Here's how the part is built. I have some questions about the finished solid (model axes, mm). A direction names the side the tool comes from. Coordinates: 2 decimals unless noted, no trailing zeros. Write each loop counter-clockwise with the first axis right and the second up, starting at its lowest first coordinate (ties: lowest second). Pieces come first, ordered by that corner, then holes.
```python
from build123d import *

# Parameters (mm, degrees)
PROFILE_R   = 2.5
PROFILE_R_2 = 1


with BuildPart() as part:
    # Tube: sweep along a curve in space
    with BuildLine() as tube_path:
        Line((-571, -44.888766616, -108.371069164), (-539.067063489, -44.888766616, -108.371069164))
        Line((-539.067063489, -44.888766616, -108.371069164), (-536.278596322, -44.805609846, -108.170310961))
        Line((-536.278596322, -44.805609846, -108.170310961), (-533.55745487, -44.558147302, -107.57288353))
        Line((-533.55745487, -44.558147302, -107.57288353), (-530.969339315, -44.152353804, -106.593211363))
        Line((-530.969339315, -44.152353804, -106.593211363), (-528.576738012, -43.598026971, -105.254948006))
        Line((-528.576738012, -43.598026971, -105.254948006), (-526.437418755, -42.908550662, -103.59040495))
        Line((-526.437418755, -42.908550662, -103.59040495), (-524.603034008, -42.100571832, -101.6397715))
        Line((-524.603034008, -42.100571832, -101.6397715), (-517.670781542, -38.519213305, -92.993607173))
        Line((-517.670781542, -38.519213305, -92.993607173), (-516.035577188, -37.409138693, -90.847413894))
        Line((-516.035577188, -37.409138693, -90.847413894), (-514.634754322, -35.896538669, -88.78294278))
        Line((-514.634754322, -35.896538669, -88.78294278), (-513.505116127, -34.021153084, -86.85443274))
        Line((-513.505116127, -34.021153084, -86.85443274), (-512.676341071, -31.832253091, -85.112550642))
        Line((-512.676341071, -31.832253091, -85.112550642), (-512.170203185, -29.387346663, -83.60306016))
        Line((-512.170203185, -29.387346663, -83.60306016), (-512, -26.750667714, -82.365619452))
        Line((-512, -26.750667714, -82.365619452), (-512, -4.999767139, -73.616976814))
        Line((-512, -4.999767139, -73.616976814), (-512.613335127, -0.677549354, -71.878495289))
        Line((-512.613335127, -0.677549354, -71.878495289), (-514.411542732, 3.350116431, -70.258488407))
        Line((-514.411542732, 3.350116431, -70.258488407), (-517.272077939, 6.808751449, -68.86735696))
        Line((-517.272077939, 6.808751449, -68.86735696), (-521, 9.462655441, -67.799904256))
        Line((-521, 9.462655441, -67.799904256), (-525.341257188, 11.130969234, -67.128875435))
        Line((-525.341257188, 11.130969234, -67.128875435), (-530, 11.7, -66.9))
        Line((-530, 11.7, -66.9), (-538.85, 11.7, -66.9))
    # Profile → Tube (sweep)
    with BuildSketch(Plane(origin=(-571, 0, 0), x_dir=(0, 0, -1), z_dir=(1, 0, 0))):
        with Locations((108.371069164, -44.888766616)):
            Circle(PROFILE_R)
        with Locations((108.371069164, -44.888766616)):
            Circle(PROFILE_R_2, mode=Mode.SUBTRACT)
    sweep(path=tube_path.line, transition=Transition.RIGHT)


solid = part.part
```
1) On a 3-axis mill with a long thin cutter (end or side, diameter ignored), from which of +Z, -Z, +X, -X, +Y, -Y can I reach the whole of each face in a straight line? I mean faces 4 (the face through (-514.59, -37.32, -89.81)), 5 (the face through (-534.406, 14.186, -66.633)). Say none if no direction works.
Values follow:
face 4: none
face 5: -X
2) Will these pins go through, and if not, where does the flat tip stop? pin 1 (5.5 mm diameter, centred on y = 13, z = -66, fed in from -X); pin 2 (10 mm diameter, centred on x = -519, y = -6, fed in from -Z); pin 3 (6 mm diameter, centred on x = -523, z = -94.5, fed in from -Y).
Values follow:
pin 1: stops at x = -538.85
pin 2: stops at z = -75.89
pin 3: stops at y = -43.04
3) We'd pull the mould along Z, two halves only. Please class faces 1 (the face through (-571, -45, -107)), 2 (the face through (-537.56, -45.23, -109.19)), 3 (the face through (-513.956, 6.719, -69.636)): pulls with the +Z half, pulls with the -Z half, needs draft (parallel to the pull), parting line crosses it, or undercut.
Values follow:
face 1: needs draft
face 2: undercut
face 3: parting line crosses it
4) Imagine slicing it at A-A on x = -549. Please give me the cut outline in (y, z).
Values follow:
outline: circle Ø5 at (-44.89, -108.37); hole circle Ø2 at (-44.89, -108.37)
5) I need wall thicknesses on probe 1 along Z at (x, y) = (-537, 11.7); probe 2 along Y at (x, z) = (-534.5, -66.9); probe 3 along Z at (x, y) = (-532, 11). Which ranges of each line are inside material? Lowest first, please.
Values follow:
probe 1: z = -69.4 to -67.9, -65.9 to -64.4
probe 2: y = 9.2 to 10.7, 12.7 to 14.2
probe 3: z = -69.3 to -67.61, -66.19 to -64.5
